from build123d import *

# Parameters (mm, degrees)
F0_R        = 67.945
F1_DEPTH    = 38.1
F2_R        = 65.405
F3_DEPTH    = 31.75
F5_W        = 2.54
F5_H        = 8.001
F7_S5_R     = 66.675
F7_T6_DEPTH = 98
F8_W        = 73.66
F8_H        = 49.022
F9_DEPTH    = 6.351
F10_W       = 85.852
F10_H       = 56.007
F11_DEPTH   = 4.826
F12_W       = 5.08
F12_H       = 53.34
F13_DEPTH   = 4.826
F14_SIZE    = 1.27
F15_W       = 1.524
F15_H       = 9.271
F16_DEPTH   = 67.946
F17_W       = 6.35
F17_H       = 5.08
F18_DEPTH   = 12.7


# Not quite as in the source:
# - a fillet or chamfer that OpenCascade refuses, or shapes differently, is made with other operations: its cross-section is extruded or revolved along the edge and cut away or added


with BuildPart() as f1:
    # F0 (on Top) → F1 (new body)
    with BuildSketch(Plane.XY):
        Circle(F0_R)
    extrude(amount=-F1_DEPTH)

    # F2 (on face) → F3 (cut)
    with BuildSketch(Plane.XY):
        Circle(F2_R)
    extrude(amount=-F3_DEPTH, mode=Mode.SUBTRACT)

    # F5 (on Front) → F6 (revolve, cut)
    with BuildSketch(Plane.XZ):
        with Locations((-67.945, -19.05)):
            Rectangle(F5_W, F5_H)
    revolve(axis=Axis((0, 0, 0), (0, 0, 1)), mode=Mode.SUBTRACT)

    # F7: chamfer of 2.54 on 1 edges, made by hand


with BuildPart() as f7_tool2:
    # F7_s3 → F7_t4 (revolve)
    with BuildSketch(Plane.XZ):
        Polygon((67.945, -12.5095), (65.405, -15.0495), (67.945, -15.0495), align=None)
    revolve(axis=Axis((0, 0, -15.0495), (0, 0, 1)))

    # F7_s5 → F7_t6 (cut, symmetric)
    with BuildSketch(Plane.XY.offset(-13.8)):
        Circle(F7_S5_R)
    extrude(amount=F7_T6_DEPTH, both=True, mode=Mode.SUBTRACT)


with BuildPart() as f1_1:
    add(f1.part)

    # F7_t1: cut F7_tool2
    add(f7_tool2.part, mode=Mode.SUBTRACT)

    # F8 (on face) → F9 (cut, through all)
    with BuildSketch(Plane.XY.offset(-31.75)):
        Rectangle(F8_W, F8_H)
    extrude(amount=-F9_DEPTH, mode=Mode.SUBTRACT)

    # F10 (on face) → F11 (cut, through all)
    with BuildSketch(Plane.XY.offset(-31.75)):
        with Locations((1.75, 0)):
            Rectangle(F10_W, F10_H)
    extrude(amount=-F11_DEPTH, mode=Mode.SUBTRACT)

    # F12 (on face) → F13 (cut, through all)
    with BuildSketch(Plane.XY.offset(-31.75)):
        with Locations((47.216, 0)):
            Rectangle(F12_W, F12_H)
    extrude(amount=-F13_DEPTH, mode=Mode.SUBTRACT)

    # F14
    f14_edges = [f1_1.edges().sort_by_distance(p)[0] for p in [
        (0, 24.511, -38.1),
        (-36.83, 0, -38.1),
        (36.83, 0, -38.1),
        (0, -24.511, -38.1),
    ]]
    chamfer(f14_edges, length=F14_SIZE)

    # F15 (on Front) → F16 (cut, through all)
    with BuildSketch(Plane.XZ):
        with Locations((-0.762, -18.415)):
            Rectangle(F15_W, F15_H)
    extrude(amount=F16_DEPTH, mode=Mode.SUBTRACT)

    # F17 (on face) → F18 (join)
    with BuildSketch(Plane.XY.offset(-31.75)):
        with Locations((-17.145, 37.465)):
            Rectangle(F17_W, F17_H)
        with Locations((34.925, 36.195)):
            Rectangle(F17_W, F17_H)
        with Locations((-15.875, -43.505)):
            Rectangle(F17_W, F17_H)
        with Locations((34.925, -38.735)):
            Rectangle(F17_W, F17_H)
    extrude(amount=F18_DEPTH)


solid = f1_1.part
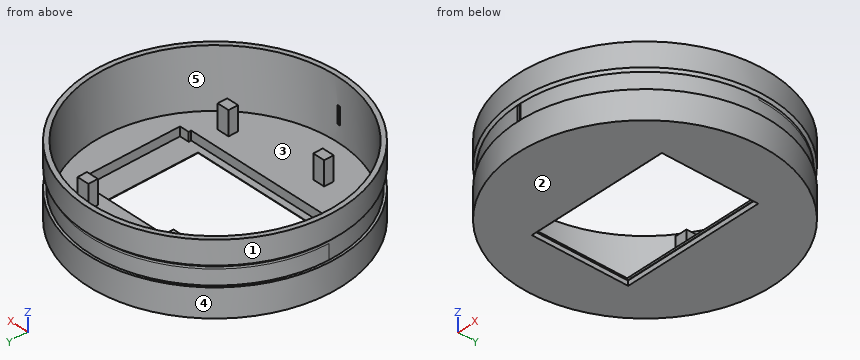
Here's how the part is built. I have some questions about the finished solid (model axes, mm). Face numbers are marked on the shaded views. A direction names the side the tool comes from. Coordinates: 2 decimals unless noted, no trailing zeros. Write each loop counter-clockwise with the first axis right and the second up, starting at its lowest first coordinate (ties: lowest second). Pieces come first, ordered by that corner, then holes. Notation, with made-up numbers: (80, -13) - (127, -13) arc R21 cw to (127, -4) - close; hole circle Ø2 at (52.5, 53.25). An arc over 180 degrees is marked (long way). Use one line per item in the form item = value.
1) Suppose I cut it at A-A, the plane z = -35. Write out the boundary of the cut face in (x, y) (1 decimal), plus the area to 3 significant figures.
Solved:
outline = circle Ø135.9 at (0, 0); hole (-41.2, -28) - (44.7, -28) - (44.7, -26.7) - (49.8, -26.7) - (49.8, 26.7) - (44.7, 26.7) - (44.7, 28) - (-41.2, 28) - close
area = 9,420 mm2
2) I'm going to push flat-ended pins straight in: P1, Ø4, axis at x = 48, z = -33.5, coming from the +Y side; P2, Ø1, axis at y = 14.5, z = -34, coming from the -X side; P3, Ø8, axis at y = 7, z = -5, coming from the +X side. Where does each tip first touch, or does it pass through?
Solved:
P1 = 50.01
P2 = -66.49
P3 = 67.88
3) I need wall thicknesses on line 1 (X direction, y = 2, z = -5.5); line 2 (Y direction, x = -1, z = -8); line 3 (Z direction, x = -41, y = -3). Which ranges of each line are inside material? Lowest first, please.
Solved:
line_1 = -67.92 to -65.37, 65.37 to 67.92
line_2 = -67.94 to -65.4, 65.4 to 67.94
line_3 = -38.1 to -36.58
4) Suppose I cut it at D-D, the plane z = -6. Write out the boundary of the cut face in (x, y) (3 decimals), plus the area to 3 significant figures.
Solved:
outline = circle Ø135.89 at (0, 0); hole circle Ø130.81 at (0, 0)
area = 1,060 mm2
5) On a 3-axis mill with a long thin cutter (end or side, diameter ignored), from which of +Z, -Z, +X, -X, +Y, -Y can I reach the whole of each face in a straight line? I mean the marked faces 4 and 5. Say none if no direction works.
Solved:
face_4 = +Z, -Z
face_5 = +Z
6) Thinking about a two-plate mould opening in Y: for the marked faces 1, 2 and 3, which applies, released by +Y, released by -Y, zero draft, split by the parting line, or undercut?
Solved:
face_1 = split by the parting line
face_2 = zero draft
face_3 = undercut
7) Suppose I cut it at C-C, the plane z = -28. Write out the boundary of the cut face in (x, y) (3 decimals), plus the area to 3 significant figures.
Solved:
outline = circle Ø135.89 at (0, 0); (-20.32, 34.925) - (-13.97, 34.925) - (-13.97, 40.005) - (-20.32, 40.005) - close; (-19.05, -46.045) - (-12.7, -46.045) - (-12.7, -40.965) - (-19.05, -40.965) - close; (31.75, -41.275) - (38.1, -41.275) - (38.1, -36.195) - (31.75, -36.195) - close; (31.75, 33.655) - (38.1, 33.655) - (38.1, 38.735) - (31.75, 38.735) - close; hole circle Ø130.81 at (0, 0)
area = 1,190 mm2
